from build123d import *

# Parameters (mm, degrees)
BOSS_EXTRUDE1_DEPTH = 20
SKETCH3_W           = 10
SKETCH3_H           = 10
CUT_EXTRUDE1_DEPTH  = 10
CIRPATTERN1_COUNT   = 4


with BuildPart() as part:
    # Sketch1 → Boss-Extrude1 (new body)
    with BuildSketch(Plane(origin=(0, 0, 0), x_dir=(1, 0, 0), z_dir=(0, 1, 0))):
        Polygon((213.546247918, 227.688383542), (227.688383542, 213.546247918), (227.688383542, -213.546247918), (213.546247918, -227.688383542), (-213.546247918, -227.688383542), (-227.688383542, -213.546247918), (-227.688383542, 213.546247918), (-213.546247918, 227.688383542), align=None)
        with BuildLine():
            Line((21.213203436, 7.071067812), (190.61731573, 176.475180106))
            ThreePointArc((190.61731573, 176.475180106), (201.515217866, 178.64290762), (207.688383542, 169.404112295))
            Line((207.688383542, 169.404112295), (207.688383542, -169.404112295))
            ThreePointArc((207.688383542, -169.404112295), (201.515217866, -178.64290762), (190.61731573, -176.475180106))
            Line((190.61731573, -176.475180106), (21.213203436, -7.071067812))
            ThreePointArc((21.213203436, -7.071067812), (18.284271247, 0), (21.213203436, 7.071067812))
        make_face(mode=Mode.SUBTRACT)
        with BuildLine():
            Line((7.071067812, -21.213203436), (176.475180106, -190.61731573))
            ThreePointArc((176.475180106, -190.61731573), (178.64290762, -201.515217866), (169.404112295, -207.688383542))
            Line((169.404112295, -207.688383542), (-169.404112295, -207.688383542))
            ThreePointArc((-169.404112295, -207.688383542), (-178.64290762, -201.515217866), (-176.475180106, -190.61731573))
            Line((-176.475180106, -190.61731573), (-7.071067812, -21.213203436))
            ThreePointArc((-7.071067812, -21.213203436), (0, -18.284271247), (7.071067812, -21.213203436))
        make_face(mode=Mode.SUBTRACT)
        with BuildLine():
            Line((-21.213203436, -7.071067812), (-190.61731573, -176.475180106))
            ThreePointArc((-190.61731573, -176.475180106), (-201.515217866, -178.64290762), (-207.688383542, -169.404112295))
            Line((-207.688383542, -169.404112295), (-207.688383542, 169.404112295))
            ThreePointArc((-207.688383542, 169.404112295), (-201.515217866, 178.64290762), (-190.61731573, 176.475180106))
            Line((-190.61731573, 176.475180106), (-21.213203436, 7.071067812))
            ThreePointArc((-21.213203436, 7.071067812), (-18.284271247, 0), (-21.213203436, -7.071067812))
        make_face(mode=Mode.SUBTRACT)
        with BuildLine():
            Line((-7.071067812, 21.213203436), (-176.475180106, 190.61731573))
            ThreePointArc((-176.475180106, 190.61731573), (-178.64290762, 201.515217866), (-169.404112295, 207.688383542))
            Line((-169.404112295, 207.688383542), (169.404112295, 207.688383542))
            ThreePointArc((169.404112295, 207.688383542), (178.64290762, 201.515217866), (176.475180106, 190.61731573))
            Line((176.475180106, 190.61731573), (7.071067812, 21.213203436))
            ThreePointArc((7.071067812, 21.213203436), (0, 18.284271247), (-7.071067812, 21.213203436))
        make_face(mode=Mode.SUBTRACT)
    extrude(amount=BOSS_EXTRUDE1_DEPTH)

    # Sketch3 → Cut-Extrude1 (cut)
    with BuildSketch(Plane(origin=(220.61731573, 0, -220.61731573), x_dir=(-0.707106781, 0, -0.707106781), z_dir=(0.707106781, 0, -0.707106781))):
        with Locations((0, 10)):
            Rectangle(SKETCH3_W, SKETCH3_H)
    cut_extrude1 = extrude(amount=-CUT_EXTRUDE1_DEPTH, mode=Mode.SUBTRACT)

    # CirPattern1: Cut-Extrude1 ×4 about axis
    cirpattern1_axis = Axis((0, 0, 0), (0, 1, 0))
    for i in range(1, CIRPATTERN1_COUNT):
        add(cut_extrude1.rotate(cirpattern1_axis, i * 360 / CIRPATTERN1_COUNT), mode=Mode.SUBTRACT)


solid = part.part
Design review of the part built by this model. Coordinates are the model's own, in mm. A direction names the side the tool comes from. Give positions to 0.01 mm unless a question says otherwise; leave off trailing zeros. Loops run counter-clockwise (first coordinate to the right, second up) from the corner with the lowest first, then second, coordinate; pieces in that order, holes last. Notation, with made-up numbers: (-14, 80.25) -> (1, 80.25) arc R28 cw to (1, 105.25) -> close; hole circle Ø2 at (45.25, 0.25). An arc over 180 degrees is marked (long way). One line per question, with ' | ' between items. Start each with the question number.
(1) We need section A-A (x = -90). State the section outline as (y, z) points, and give its area (3 significant figures).
(2) We need section B-B (z = 78). State the section outline as (x, y) points.
(3) For line 1 (X direction, y = 16.25, z = 7.5); line 2 (Z direction, x = 132.5, y = 4.75); line 3 (X direction, y = 15.5, z = 17), list the stretches that pass through material, from the lowest coordinate up.
(4) We need section C-C (y = 11.75). State how many separate pieces and enclosed holes the cut face has, and give its area (3 significant figures).
(5) Draft analysis for pull direction Y (two halves, no side actions). For faces 1 (the face through (-227.688, 10, 3)), 2 (the face through (-217, 15, -217)), state which applies: +Y half, -Y half, draft (parallel to the pull), parting line (faces both ways), or undercut.
(6) For faces 3 (the face through (-220.518, 3.193, 220.716)), 4 (the face through (92.96, 9.86, -107.1)), 5 (the face through (217, 15, 217)), list the 3-axis set-ups (+Z, -Z, +X, -X, +Y, -Y) from which the entire face can be reached by the end or side of a thin tool; tool diameter is ignored.
The answers:
1) outline: (0, -227.69) -> (20, -227.69) -> (20, -207.69) -> (0, -207.69) -> close; (0, -104.14) -> (20, -104.14) -> (20, -75.86) -> (0, -75.86) -> close; (0, 75.86) -> (20, 75.86) -> (20, 104.14) -> (0, 104.14) -> close; (0, 207.69) -> (20, 207.69) -> (20, 227.69) -> (0, 227.69) -> close | area: 1,930 mm^2
2) outline: (-227.69, 0) -> (-207.69, 0) -> (-207.69, 20) -> (-227.69, 20) -> close; (-92.14, 0) -> (-63.86, 0) -> (-63.86, 20) -> (-92.14, 20) -> close; (63.86, 0) -> (92.14, 0) -> (92.14, 20) -> (63.86, 20) -> close; (207.69, 0) -> (227.69, 0) -> (227.69, 20) -> (207.69, 20) -> close
3) line 1: x = -227.69 to -207.69, -21.64 to 21.64, 207.69 to 227.69 | line 2: z = -227.69 to -207.69, -146.64 to -118.36, 118.36 to 146.64, 207.69 to 227.69 | line 3: x = -227.69 to -207.69, -31.14 to 31.14, 207.69 to 227.69
4) separate pieces: 1 | enclosed holes: 4 | area: 57,800 mm^2
5) face 1: draft | face 2: undercut
6) face 3: +Z, -X, +Y, -Y | face 4: +Y, -Y | face 5: none
